from build123d import *

# Parameters (mm, degrees)
ESQUISSE1_W             = 180
ESQUISSE1_H             = 80
BOSS_EXTRU_1_DEPTH      = 5
ESQUISSE2_R             = 0.9
ENL_V_MAT_EXTRU_1_DEPTH = 5
ESQUISSE4_R             = 0.9
ENL_V_MAT_EXTRU_2_DEPTH = 99.615414617
ESQUISSE5_R             = 1.2
ENL_V_MAT_EXTRU_3_DEPTH = 99.615414617
ESQUISSE6_W             = 98.043134308
ESQUISSE6_H             = 36.477445857
ENL_V_MAT_EXTRU_4_DEPTH = 99.615414617


with BuildPart() as part:
    # Esquisse1 → Boss.-Extru.1 (new body)
    with BuildSketch(Plane.XY):
        Rectangle(ESQUISSE1_W, ESQUISSE1_H)
    extrude(amount=BOSS_EXTRU_1_DEPTH)

    # Esquisse2 → Enlèv. mat.-Extru.1 (cut)
    with BuildSketch(Plane(origin=(0, 0, 0), x_dir=(-1, 0, 0), z_dir=(0, 0, -1))):
        with Locations((-46.756409802, 32.95183049)):
            Circle(ESQUISSE2_R)
        with Locations((-9.456409802, 32.95183049)):
            Circle(ESQUISSE2_R)
        with Locations((0.543590198, 32.95183049)):
            Circle(ESQUISSE2_R)
        with Locations((37.843590198, 32.95183049)):
            Circle(ESQUISSE2_R)
        with Locations((-46.756409802, 12.75183049)):
            Circle(ESQUISSE2_R)
        with Locations((-9.456409802, 12.75183049)):
            Circle(ESQUISSE2_R)
        with Locations((0.543590198, 12.75183049)):
            Circle(ESQUISSE2_R)
        with Locations((37.843590198, 12.75183049)):
            Circle(ESQUISSE2_R)
        with Locations((-46.756409802, -7.44816951)):
            Circle(ESQUISSE2_R)
        with Locations((-9.456409802, -7.44816951)):
            Circle(ESQUISSE2_R)
        with Locations((0.543590198, -7.44816951)):
            Circle(ESQUISSE2_R)
        with Locations((37.843590198, -7.44816951)):
            Circle(ESQUISSE2_R)
    extrude(amount=-ENL_V_MAT_EXTRU_1_DEPTH, mode=Mode.SUBTRACT)

    # Esquisse4 → Enlèv. mat.-Extru.2 (cut, through all)
    with BuildSketch(Plane(origin=(0, 0, 0), x_dir=(-1, 0, 0), z_dir=(0, 0, -1))):
        with Locations((85.5, 0)):
            Circle(ESQUISSE4_R)
        with Locations((77.5, 0)):
            Circle(ESQUISSE4_R)
        with Locations((69.5, 0)):
            Circle(ESQUISSE4_R)
        with Locations((77.5, 8)):
            Circle(ESQUISSE4_R)
        with Locations((69.5, 8)):
            Circle(ESQUISSE4_R)
        with Locations((85.5, 8)):
            Circle(ESQUISSE4_R)
        with Locations((69.5, -8)):
            Circle(ESQUISSE4_R)
        with Locations((77.5, -8)):
            Circle(ESQUISSE4_R)
        with Locations((85.5, -8)):
            Circle(ESQUISSE4_R)
        with Locations((-24.5, 0)):
            Circle(ESQUISSE4_R)
        with Locations((-32.5, 0)):
            Circle(ESQUISSE4_R)
        with Locations((-40.5, 0)):
            Circle(ESQUISSE4_R)
        with Locations((-32.5, 8)):
            Circle(ESQUISSE4_R)
        with Locations((-40.5, 8)):
            Circle(ESQUISSE4_R)
        with Locations((-24.5, 8)):
            Circle(ESQUISSE4_R)
        with Locations((-40.5, -8)):
            Circle(ESQUISSE4_R)
        with Locations((-32.5, -8)):
            Circle(ESQUISSE4_R)
        with Locations((-24.5, -8)):
            Circle(ESQUISSE4_R)
    extrude(amount=-ENL_V_MAT_EXTRU_2_DEPTH, mode=Mode.SUBTRACT)

    # Esquisse5 → Enlèv. mat.-Extru.3 (cut, through all)
    with BuildSketch(Plane(origin=(0, 0, 0), x_dir=(-1, 0, 0), z_dir=(0, 0, -1))):
        with Locations((-60, 14.8)):
            Circle(ESQUISSE5_R)
        with Locations((-86, 14.8)):
            Circle(ESQUISSE5_R)
        with Locations(Location((-86, -17.1, 0), (0, 0, 180))):
            Circle(ESQUISSE5_R)
        with Locations(Location((-60, -17.1, 0), (0, 0, 180))):
            Circle(ESQUISSE5_R)
        with Locations((67.75, 14.8)):
            Circle(ESQUISSE5_R)
        with Locations((41.75, 14.8)):
            Circle(ESQUISSE5_R)
        with Locations(Location((41.75, -17.1, 0), (0, 0, 180))):
            Circle(ESQUISSE5_R)
        with Locations(Location((67.75, -17.1, 0), (0, 0, 180))):
            Circle(ESQUISSE5_R)
    extrude(amount=-ENL_V_MAT_EXTRU_3_DEPTH, mode=Mode.SUBTRACT)

    # Esquisse6 → Enlèv. mat.-Extru.4 (cut, through all)
    with BuildSketch(Plane(origin=(0, 0, 0), x_dir=(-1, 0, 0), z_dir=(0, 0, -1))):
        with Locations((-4.148056784, 12.955156499)):
            Rectangle(ESQUISSE6_W, ESQUISSE6_H)
    extrude(amount=-ENL_V_MAT_EXTRU_4_DEPTH, mode=Mode.SUBTRACT)


solid = part.part
Check sheet for the modelled part. Datum: model origin and axes. Units: mm. A direction names the side the tool comes from. Give positions to 0.01 mm unless a question says otherwise; leave off trailing zeros. Write each loop counter-clockwise with the first axis right and the second up, starting at its lowest first coordinate (ties: lowest second). Pieces come first, ordered by that corner, then holes. Notation, with made-up numbers: (37, 80) -> (61, 80) arc R14 cw to (61, 85) -> close; hole circle Ø4 at (53.25, 51.5). An arc over 180 degrees is marked (long way). Use one line per item in the form item = value. Start each with the question number.
1. Section check A-A (x = 15). Record the cut outline in (y, z).
2. Mould release check, pull along X, two halves, no side actions. Record for faces 1 (the flat face through (90, -1, 2)), 2 (the flat face through (-90, -1, 2)), 3 (the flat face through (53.17, 13, 2)): pulls with the +X half, pulls with the -X half, needs draft (parallel to the pull), parting line crosses it, or undercut.
3. Section check B-B (z = 2.55). Count the separate pieces of the cut face and the enclosed holes in it, and give its area (3 significant figures).
4. Thickness scan on line 1 along X through (y, z) = (-17.1, 2.75); line 2 along Y through (x, z) = (-69.5, 1); line 3 along Y through (x, z) = (39, 1.8). Record the ranges inside material, lowest first. Write a range as from..to.
5. Access from +Z, -Z, +X, -X, +Y, -Y to the whole of each face (thin tool, end or side, straight path). Record for faces 4 (the flat face through (5, 31.194, 2)), 5 (the flat face through (-1.3, -8.3, 5)).
Conclusion:
q1.outline = (-40, 0) -> (-5.28, 0) -> (-5.28, 5) -> (-40, 5) -> close; (31.19, 0) -> (40, 0) -> (40, 5) -> (31.19, 5) -> close
q2.face_1 = pulls with the +X half
q2.face_2 = pulls with the -X half
q2.face_3 = undercut
q3.separate_pieces = 1
q3.enclosed_holes = 28
q3.area = 10,700 mm²
q4.line_1 = -90..-68.95, -66.55..-42.95, -40.55..58.8, 61.2..84.8, 87.2..90
q4.line_2 = -40..-8.9, -7.1..-0.9, 0.9..7.1, 8.9..40
q4.line_3 = -40..-5.28, 31.19..40
q5.face_4 = +Z, -Z
q5.face_5 = +Z, +X, -X, +Y, -Y
